from build123d import *

# Parameters (mm, degrees)
F0_R          = 10
F1_DEPTH      = 25
F1_DEPTH_BACK = 25


with BuildPart() as f1:
    # F0 (on Top) → F1 (new body, two sides)
    with BuildSketch(Plane.XY) as f1_sk:
        with BuildLine():
            Line((-40, 20), (40, 20))
            Line((40, 20), (40, 110))
            Line((40, 110), (30, 110))
            ThreePointArc((30, 110), (0, 80), (-30, 110))
            Line((-30, 110), (-40, 110))
            Line((-40, 110), (-40, 20))
        make_face()
        with BuildLine():
            Line((30, -110), (40, -110))
            Line((40, -110), (40, -20))
            Line((40, -20), (-40, -20))
            Line((-40, -20), (-40, -110))
            Line((-40, -110), (-30, -110))
            ThreePointArc((-30, -110), (0, -80), (30, -110))
        make_face()
        with BuildLine():
            Line((-40, -20), (40, -20))
            ThreePointArc((40, -20), (20, 0), (40, 20))
            Line((40, 20), (-40, 20))
            ThreePointArc((-40, 20), (-20, 0), (-40, -20))
        make_face()
        Circle(F0_R, mode=Mode.SUBTRACT)
    extrude(amount=F1_DEPTH)
    extrude(f1_sk.sketch, amount=-F1_DEPTH_BACK)


solid = f1.part
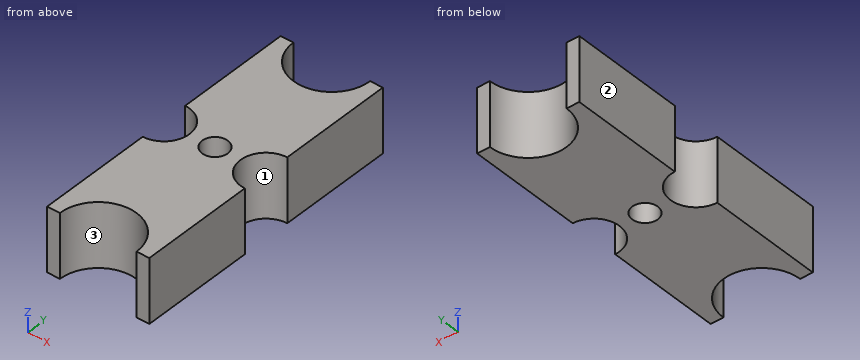
The model under review builds one solid part; all positions refer to its coordinate system, in mm. Face numbers are marked on the shaded views. Give positions to 0.01 mm unless a question says otherwise; leave off trailing zeros. Write each loop counter-clockwise with the first axis right and the second up, starting at its lowest first coordinate (ties: lowest second). Pieces come first, ordered by that corner, then holes.
1. Add section C-C, the plane z = 20.5. Write out the cut boundary in (x, y), plus the area to 3 significant figures.
2. For P1, Ø5, axis at x = 9, z = -17, coming from the +Y side; P2, Ø8, axis at x = -6, z = 9.5, coming from the +Y side; P3, Ø10, axis at y = 7.5, z = 4.5, coming from the -X side, all flat-tipped, find the tip position at first contact; note any pin that passes through.
3. Wall thickness on L1, parallel to Y at x = 0, z = 3.5; L2, parallel to Y at x = 32, z = -3.5; L3, parallel to X at y = 1, z = -7: over which ranges is each line inside the solid? List them lowest first.
4. Draft analysis for pull direction X (two halves, no side actions). For the marked faces 1, 2 and 3, state which applies: +X half, -X half, draft (parallel to the pull), parting line (faces both ways), or undercut.
5. Add section B-B, the plane y = 0. Write out the cut boundary in (x, z), plus the area to 3 significant figures.
6. Add section A-A, the plane x = 0. Write out the cut boundary in (y, z).
Worked answers:
1. outline: (-40, -110) - (-30, -110) arc R30 cw to (30, -110) - (40, -110) - (40, -20) arc R20 cw to (40, 20) - (40, 110) - (30, 110) arc R30 cw to (-30, 110) - (-40, 110) - (-40, 20) arc R20 cw to (-40, -20) - close; hole circle Ø20 at (0, 0)
1. area: 13,200 mm2
2. P1: stops at y = 82.29
2. P2: stops at y = 81.72
2. P3: stops at x = -24.39
3. L1: y = -80 to -10, 10 to 80
3. L2: y = -110 to -18.33, 18.33 to 110
3. L3: x = -20.03 to -9.95, 9.95 to 20.03
4. face 1: +X half
4. face 2: -X half
4. face 3: undercut
5. outline: (-20, -25) - (-10, -25) - (-10, 25) - (-20, 25) - close; (10, -25) - (20, -25) - (20, 25) - (10, 25) - close
5. area: 1,000 mm2
6. outline: (-80, -25) - (-10, -25) - (-10, 25) - (-80, 25) - close; (10, -25) - (80, -25) - (80, 25) - (10, 25) - close
